Answer from the drawing. Dimensions are ordinates in mm from the lowest x, y and z of the part. A direction names the side the tool comes from. Give positions to 0.01 mm unless a question says otherwise; leave off trailing zeros. Loops run counter-clockwise (first coordinate to the right, second up) from the corner with the lowest first, then second, coordinate; pieces in that order, holes last.
Item 1: Section C-C, the plane y = 17.5 is taken. Give the vertices of the cut face in (x, z), and give its area (3 significant figures).
Item 2: A tool of negligible diameter and unlimited length cuts with its end or side. For the marked faces 1 and 2, from which of +Z, -Z, +X, -X, +Y, -Y can it reach the whole face along a straight path? Write none if from no direction.
Item 3: Consider line 1 along Z through (x, y) = (13.5, 25.75). Determine where the line is inside the solid, lowest interval first.
Item 4: Section A-A, the plane z = 2.05 is taken. Give the vertices of the cut face in (x, y).
Item 5: Section B-B, the plane x = 20.25 is taken. Give the vertices of the cut face in (y, z).
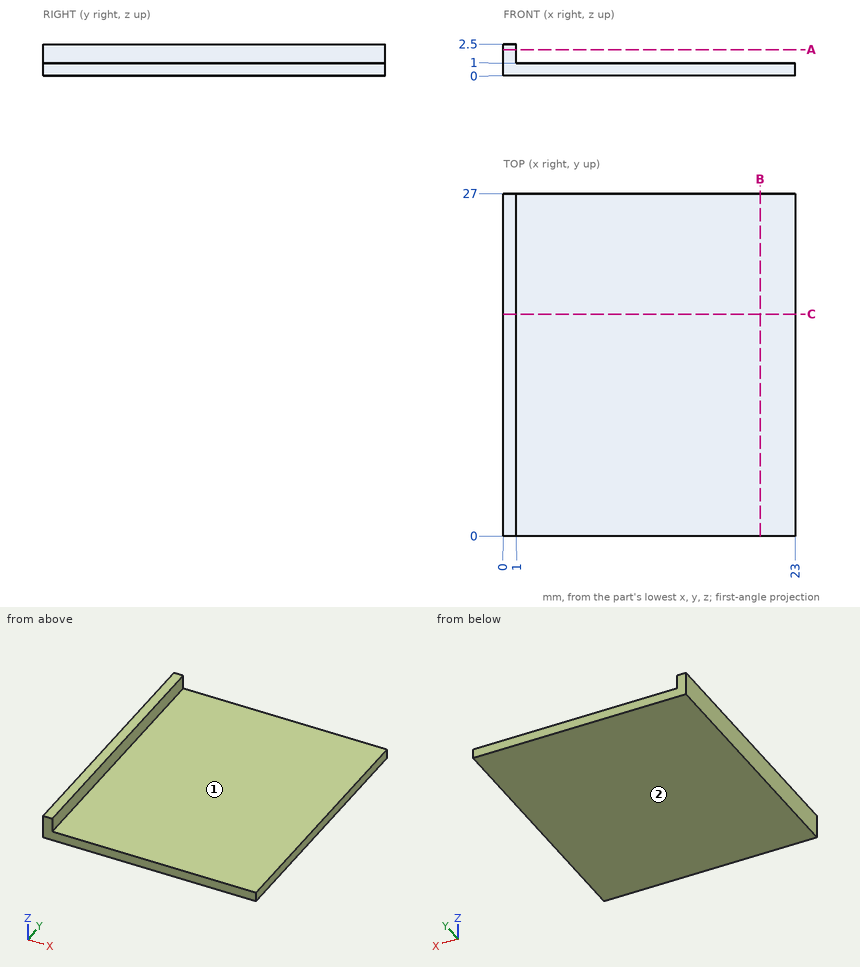
Worked answers:
1. outline: (0, 0) - (23, 0) - (23, 1) - (1, 1) - (1, 2.5) - (0, 2.5) - close
1. area: 24.5 mm2
2. face 1: +Z, +X, +Y, -Y
2. face 2: -Z, +X, -X, +Y, -Y
3. line 1: z = 0 to 1
4. outline: (0, 0) - (1, 0) - (1, 27) - (0, 27) - close
5. outline: (0, 0) - (27, 0) - (27, 1) - (0, 1) - close
